```python
from build123d import *

# Parameters (mm, degrees)
SKETCH2_W           = 10
SKETCH2_H           = 100
SKETCH2_W_2         = 80
SKETCH2_H_2         = 5
BOSS_EXTRUDE2_DEPTH = 160
FILLET1_R           = 20
SKETCH3_R           = 5
CUT_EXTRUDE2_DEPTH  = 10


with BuildPart() as part:
    # Sketch2 → Boss-Extrude2 (new body)
    with BuildSketch(Plane.XY):
        with Locations((40, 50)):
            Rectangle(SKETCH2_W, SKETCH2_H)
        with Locations((40, -2.5)):
            Rectangle(SKETCH2_W_2, SKETCH2_H_2)
    extrude(amount=BOSS_EXTRUDE2_DEPTH)

    # Fillet1
    fillet1_edges = [part.edges().sort_by_distance(p)[0] for p in [
        (45, 0, 80),
        (35, 0, 80),
    ]]
    fillet(fillet1_edges, radius=FILLET1_R)

    # Sketch3 → Cut-Extrude2 (cut)
    with BuildSketch(Plane(origin=(0, 0, 0), x_dir=(1, 0, 0), z_dir=(0, 1, 0))):
        with Locations((72.5, -20)):
            Circle(SKETCH3_R)
        with Locations((72.5, -140)):
            Circle(SKETCH3_R)
        with Locations((7.5, -140)):
            Circle(SKETCH3_R)
        with Locations((7.5, -20)):
            Circle(SKETCH3_R)
    extrude(amount=-CUT_EXTRUDE2_DEPTH, mode=Mode.SUBTRACT)


solid = part.part
```
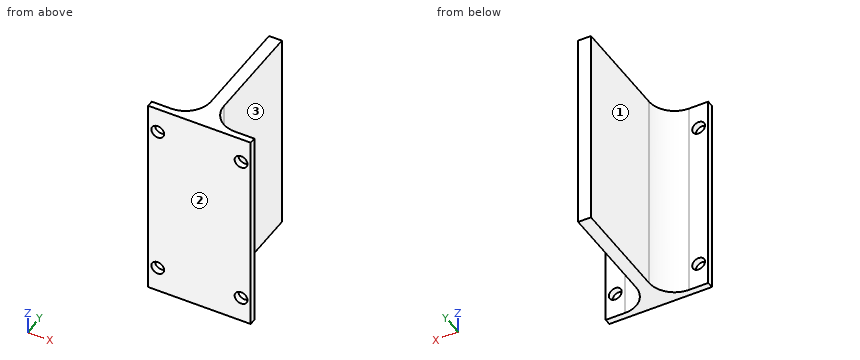
CAD build for the part. Positions are in the model's coordinates, mm. Face numbers are marked on the shaded views. A direction names the side the tool comes from. Round coordinates to 2 decimals unless told otherwise and drop trailing zeros. Loops run counter-clockwise (first coordinate to the right, second up) from the corner with the lowest first, then second, coordinate; pieces in that order, holes last. Notation, with made-up numbers: M 4.25,53.5 L 20.25,53.5 A22 ccw 20.25,64.5 Z; hole C 77,40 d5. An arc over 180 degrees is marked long. Return JSON: item names as keys, results as strings. Group by question number.
(1) Saw through at C-C, the plane z = 42.5. List the corners of the cut face in (x, y).
(2) Saw through at D-D, the plane x = 6. List the corners of the cut face in (y, z).
(3) Saw through at A-A, the plane z = 20. List the corners of the cut face in (x, y), and give its area (3 significant figures).
(4) Wall check: probe 1 along X at (y, z) = (-2.8, 140); probe 2 along Z at (x, y) = (72.5, -1.8); probe 3 along X at (y, z) = (27.5, 104). Give the ranges that are in metal, low to high. Write a range as [from, to].
(5) Tool access for the marked faces 1, 2 and 3: list every direction of +Z, -Z, +X, -X, +Y, -Y with a clear straight run to the whole face (end or side of a thin tool).
(6) Saw through at B-B, the plane x = 72.5. List the corners of the cut face in (y, z).
(7) Drop flat-ended pins along their axis: P1, Ø5, axis at y = 29, z = 22, coming from the -X side; P2, Ø12, axis at x = 76, z = 108, coming from the +Y side; P3, Ø24, axis at y = 71, z = 48.5, coming from the +X side. Give the stop position or say it passes through.
Answer list:
{
 "1": {"outline": "M 0,-5 L 80,-5 L 80,0 L 65,0 A20 cw 45,20 L 45,100 L 35,100 L 35,20 A20 cw 15,0 L 0,0 Z"},
 "2": {"outline": "M -5,0 L 0,0 L 0,15.23 L -5,15.23 Z; M -5,24.77 L 0,24.77 L 0,135.23 L -5,135.23 Z; M -5,144.77 L 0,144.77 L 0,160 L -5,160 Z"},
 "3": {"outline": "M 0,-5 L 2.5,-5 L 2.5,0 L 0,0 Z; M 12.5,-5 L 67.5,-5 L 67.5,0 L 65,0 A20 cw 45,20 L 45,100 L 35,100 L 35,20 A20 cw 15,0 L 12.5,0 Z; M 77.5,-5 L 80,-5 L 80,0 L 77.5,0 Z", "area": "1,470 mm2"},
 "4": {"probe 1": "[0, 2.5], [12.5, 67.5], [77.5, 80]", "probe 2": "[0, 15], [25, 135], [145, 160]", "probe 3": "[35, 45]"},
 "5": {"face 1": "+Z, -Z, -X, +Y", "face 2": "+Z, -Z, +X, -X, -Y", "face 3": "+Z, -Z, +X, +Y"},
 "6": {"outline": "M -5,0 L 0,0 L 0,15 L -5,15 Z; M -5,25 L 0,25 L 0,135 L -5,135 Z; M -5,145 L 0,145 L 0,160 L -5,160 Z"},
 "7": {"P1": "x = 35", "P2": "y = 0", "P3": "x = 45"}
}
